```python
from build123d import *

# Parameters (mm, degrees)
SKETCH_2_R               = 3.3
BASE_PLATE_M6_DEPTH      = 198.301799282
PATTERN_CIRCULAR_1_COUNT = 8


with BuildPart() as part:
    # ｽｹｯﾁ1 → 回転1 (revolve)
    with BuildSketch(Plane.XY, mode=Mode.PRIVATE) as revolve_1_sk:
        Polygon((-109.5, 26.845447074), (-136, 26.845447074), (-136, 20.845447074), (-112.5, 20.845447074), (-112.5, -14.154552926), (-119.5, -21.154552926), (-119.5, -23.154552926), (-110, -23.154552926), (-104, -17.154552926), (-67.5, -17.154552926), (-67.5, -11.154552926), (-109.5, -11.154552926), align=None)
    revolve(revolve_1_sk.sketch.rotate(Axis((0, 100.817249739, 0), (0, -1, 0)), 270), axis=Axis((0, 100.817249739, 0), (0, -1, 0)))

    # ｽｹｯﾁ2 → Base_Plateへの固定用穴(M6の六角ボルトを使用) (cut, through all)
    with BuildSketch(Plane.XZ.offset(-20.845447074)):
        with Locations(Location((123, 0, 0), (0, 0, 270))):
            Circle(SKETCH_2_R)
    base_plate_m6 = extrude(amount=-BASE_PLATE_M6_DEPTH, mode=Mode.SUBTRACT)

    # 円形ﾊﾟﾀｰﾝ1: Base_Plateへの固定用穴(M6の六角ボルトを使用) ×8 about axis
    pattern_circular_1_axis = Axis((0, 0, 0), (0, 1, 0))
    for i in range(1, PATTERN_CIRCULAR_1_COUNT):
        add(base_plate_m6.rotate(pattern_circular_1_axis, i * 360 / PATTERN_CIRCULAR_1_COUNT), mode=Mode.SUBTRACT)


solid = part.part
```
Can you work these out from the model? Positions are in its coordinate system, mm. A direction names the side the tool comes from. Coordinates: 2 decimals unless noted, no trailing zeros. Loops run counter-clockwise (first coordinate to the right, second up) from the corner with the lowest first, then second, coordinate; pieces in that order, holes last. Notation, with made-up numbers: (72, -4.5) - (107, -4.5) arc R15 ccw to (107, 17.5) - close; hole circle Ø4 at (3.5, -34). An arc over 180 degrees is marked (long way). Answer as CSV lines item,"result". Start each with the question number.
1) I need wall thicknesses on line 1 (X direction, y = 23, z = 0); line 2 (X direction, y = -13, z = 0); line 3 (X direction, y = 9.5, z = 2). Which ranges of each line are inside material? Lowest first, please. Write a range as from..to.
2) For pin 1 (4 mm diameter, centred on y = 13, z = 15, fed in from +X); pin 2 (12 mm diameter, centred on y = -7, z = -40, fed in from +X); pin 3 (1.5 mm diameter, centred on x = -16, y = -15, fed in from -Z); pin 4 (4 mm diameter, centred on x = -86.97, z = -86.97, fed in from +Y), each with a flat end and sliding along its axis, tell me the tip position at first contact or that it passes through.
3) Suppose I cut it at A-A (z = 0). Count the separate pieces of the cut face and the enclosed holes in it, plus the area to 3 significant figures.
4) Thinking about a two-plate mould opening in Z: for faces 6 (the cylindrical face through (45.769, -22.169, 110.388)), 7 (the flat face through (110, 26.845, 1)), 8 (the conical face through (-31.33, -17.45, 99.48)), which applies, pulls with the +Z half, pulls with the -Z half, needs draft (parallel to the pull), parting line crosses it, or undercut?
5) Suppose I cut it at C-C (z = -123). Please give me the cut outline in (x, y), plus the area to 3 significant figures.
6) Suppose I cut it at D-D (y = 1.5). Please give me the cut outline in (x, z).
7) Which directions (+Z, -Z, +X, -X, +Y, -Y) give clear straight access to the entire face, cutting with the end or side of a thin tool? Please do faces 1 (the cylindrical face through (106.896, 8.111, -23.737)), 2 (the flat face through (68, -17.155, -1)), 3 (the cylindrical face through (-83.925, 23.803, 88.236)), 4 (the flat face through (97, -23.155, 53)), 5 (the cylindrical face through (-4.95, 3.1, -112.39)).
Check result:
1,line 1,"x = -136..-126.3, -119.7..-109.5, 109.5..119.7, 126.3..136"
1,line 2,"x = -112.5..-67.5, 67.5..112.5"
1,line 3,"x = -112.48..-109.48, 109.48..112.48"
2,pin 1,"stops at x = 111.75"
2,pin 2,"stops at x = 107.24"
2,pin 3,"stops at z = -112.98"
2,pin 4,"passes through"
3,separate pieces,"4"
3,enclosed holes,"0"
3,area,"1,110 mm²"
4,face 6,"parting line crosses it"
4,face 7,"needs draft"
4,face 8,"undercut"
5,outline,"(-58.03, 20.85) - (-3.3, 20.85) - (-3.3, 26.85) - (-58.03, 26.85) - close; (3.3, 20.85) - (58.03, 20.85) - (58.03, 26.85) - (3.3, 26.85) - close"
5,area,"657 mm²"
6,outline,"circle Ø225 at (0, 0); hole circle Ø219 at (0, 0)"
7,face 1,"+Y"
7,face 2,"-Y"
7,face 3,"+Y, -Y"
7,face 4,"+Z, -Z, +X, -X, -Y"
7,face 5,"none"
